Could you check a few things on this model? Use its own coordinates, in mm. A direction names the side the tool comes from. Coordinates: 2 decimals unless noted, no trailing zeros. Write each loop counter-clockwise with the first axis right and the second up, starting at its lowest first coordinate (ties: lowest second). Pieces come first, ordered by that corner, then holes. Notation, with made-up numbers: (38.5, 75.25) - (72.5, 75.25) arc R24 ccw to (72.5, 114.25) - close; hole circle Ø1 at (-19.5, 57.25). An arc over 180 degrees is marked (long way). Answer as a JSON object with one key per item and string values. Group by question number.
1) Please list where these lines run through material, in increasing order: line 1 along X through (y, z) = (9, 4.5); line 2 along Y through (x, z) = (-39, 5); line 3 along X through (y, z) = (28, 5.75).
2) Will these pins go through, and if not, where does the flat tip stop? pin 1 Ø3 at (x, z) = (27.5, 3.5) entering from -Y; pin 2 Ø1.5 at (x, z) = (4.5, 5.5) entering from -Y; pin 3 Ø2 at (x, z) = (-50.5, 4.5) entering from -Y.
3) We'd pull the mould along X, two halves only. Please class faces 1 (the flat face through (-42.925, 16.15, 3.381)), 2 (the cylindrical face through (-18.508, -19.591, 3.381)), 3 (the flat face through (-6.503, 10.585, 3.381)), 4 (the flat face through (42.925, -16.15, 3.381)): released by +X, released by -X, zero draft, split by the parting line, or undercut.
4) On a 3-axis mill with a long thin cutter (end or side, diameter ignored), from which of +Z, -Z, +X, -X, +Y, -Y can I reach the whole of each face in a straight line? I mean faces 5 (the cylindrical face through (-18.42, 19.23, 3.38)), 6 (the flat face through (6.61, 10.56, 3.38)), 7 (the flat face through (-6.78, -10.394, 3.381)). Say none if no direction works.
5) If we section it at A-A (x = 0): Write out the boundary of the cut face in (y, z).
6) If we section it at C-C (z = 2.25): Write out the boundary of the cut face in (x, y).
7) If we section it at D-D (y = 3.5): Write out the boundary of the cut face in (x, z), plus the area to 3 significant figures.
8) If we section it at B-B (y = -25): Write out the boundary of the cut face in (x, z), plus the area to 3 significant figures.
```python
from build123d import *

# Parameters (mm, degrees)
F0_R     = 9.744375
F1_DEPTH = 6.858


with BuildPart() as f1:
    # F0 (on Top) → F1 (new body)
    with BuildSketch(Plane.XY):
        with BuildLine():
            Line((-10.271028, -9.6542), (-10.271028, -9.41727))
            Line((-10.271028, -9.41727), (-3.189457, -11.398748))
            ThreePointArc((-3.189457, -11.398748), (-0.855809, -11.805579), (1.512117, -11.739574))
            Line((1.512117, -11.739574), (3.940298, -11.161458))
            Line((3.940298, -11.161458), (10.271028, -9.6542))
            ThreePointArc((10.271028, -9.6542), (18.465013, -19.411145), (15.724788, -31.854236))
            Line((15.724788, -31.854236), (70.897943, 0))
            Line((70.897943, 0), (15.724788, 31.854236))
            ThreePointArc((15.724788, 31.854236), (18.465013, 19.411145), (10.271028, 9.6542))
            Line((10.271028, 9.6542), (2.839986, 11.490804))
            ThreePointArc((2.839986, 11.490804), (0, 11.836558), (-2.839986, 11.490804))
            Line((-2.839986, 11.490804), (-10.271028, 9.6542))
            ThreePointArc((-10.271028, 9.6542), (-18.465013, 19.411145), (-15.724788, 31.854236))
            Line((-15.724788, 31.854236), (-70.897943, 0))
            Line((-70.897943, 0), (-15.724788, -31.854236))
            ThreePointArc((-15.724788, -31.854236), (-18.465013, -19.411145), (-10.271028, -9.6542))
        make_face()
        with Locations((-45.329779, 0)):
            Circle(F0_R, mode=Mode.SUBTRACT)
        with BuildLine():
            ThreePointArc((-6.35, 0), (0, 6.35), (6.35, 0))
            ThreePointArc((6.35, 0), (0, -6.35), (-6.35, 0))
        make_face(mode=Mode.SUBTRACT)
        with BuildLine():
            ThreePointArc((55.074155, 0), (45.329779, -9.744375), (35.585404, 0))
            ThreePointArc((35.585404, 0), (45.329779, 9.744375), (55.074155, 0))
        make_face(mode=Mode.SUBTRACT)
    extrude(amount=F1_DEPTH)


solid = f1.part
```
Here are the results:
{
 "1": {"line 1": "x = -55.31 to -49.07, -41.59 to 41.59, 49.07 to 55.31", "line 2": "y = -18.42 to -7.41, 7.41 to 18.42", "line 3": "x = -22.4 to -17.93, 17.93 to 22.4"},
 "2": {"pin 1": "stops at y = -25.92", "pin 2": "stops at y = -11.21", "pin 3": "stops at y = -12.35"},
 "3": {"face 1": "released by -X", "face 2": "undercut", "face 3": "undercut", "face 4": "released by +X"},
 "4": {"face 5": "+Z, -Z", "face 6": "+Z, -Z, +Y", "face 7": "+Z, -Z, -Y"},
 "5": {"outline": "(-11.84, 0) - (-6.35, 0) - (-6.35, 6.86) - (-11.84, 6.86) - close; (6.35, 0) - (11.84, 0) - (11.84, 6.86) - (6.35, 6.86) - close"},
 "6": {"outline": "(-70.9, 0) - (-15.72, -31.85) arc R14.42 cw to (-10.27, -9.65) - (-10.27, -9.42) - (-3.19, -11.4) arc R11.84 ccw to (1.51, -11.74) - (10.27, -9.65) arc R14.42 cw to (15.72, -31.85) - (70.9, 0) - (15.72, 31.85) arc R14.42 cw to (10.27, 9.65) - (2.84, 11.49) arc R11.84 ccw to (-2.84, 11.49) - (-10.27, 9.65) arc R14.42 cw to (-15.72, 31.85) - close; hole circle Ø19.49 at (-45.33, 0); hole circle Ø12.7 at (0, 0); hole circle Ø19.49 at (45.33, 0)"},
 "7": {"outline": "(-64.84, 0) - (-54.42, 0) - (-54.42, 6.86) - (-64.84, 6.86) - close; (-36.24, 0) - (-5.3, 0) - (-5.3, 6.86) - (-36.24, 6.86) - close; (5.3, 0) - (36.24, 0) - (36.24, 6.86) - (5.3, 6.86) - close; (54.42, 0) - (64.84, 0) - (64.84, 6.86) - (54.42, 6.86) - close", "area": "567 mm²"},
 "8": {"outline": "(-27.6, 0) - (-18.72, 0) - (-18.72, 6.86) - (-27.6, 6.86) - close; (18.72, 0) - (27.6, 0) - (27.6, 6.86) - (18.72, 6.86) - close", "area": "122 mm²"}
}
